Source: CAD feature listing. Evaluate the final solid. Frame: model axes, mm. A direction names the side the tool comes from. Round coordinates to 2 decimals unless told otherwise and drop trailing zeros. Order: outer loops, then holes, each group sorted by start corner. A loop starts at its lowest first (then second) coordinate and runs counter-clockwise, first axis right, second up. Notation, with made-up numbers: (-33.75, -22) -> (-5.75, -22) arc R17 cw to (-5.75, -6) -> close; hole circle Ø4 at (41, 44.5). An arc over 180 degrees is marked (long way). Use a Markdown table: item, result. Add a question column.
```python
from build123d import *

# Parameters (mm, degrees)
SKETCH_1_R               = 8
EXTRUDE_1_DEPTH          = 180
SKETCH_2_R               = 4
CUT_EXTRUDE_1_DEPTH      = 9
CUT_EXTRUDE_1_DEPTH_BACK = 9
SKETCH_3_OUTSIDE_W       = 54.284
SKETCH_3_OUTSIDE_H       = 54.284
SKETCH_3_OUTSIDE_W_2     = 8
SKETCH_3_OUTSIDE_H_2     = 20
CUT_EXTRUDE_2_DEPTH      = 20


with BuildPart() as part:
    # 草图1 → 凸台-拉伸1 (new body)
    with BuildSketch(Plane(origin=(0, 0, 0), x_dir=(0, 0, -1), z_dir=(1, 0, 0))):
        Circle(SKETCH_1_R)
    extrude(amount=EXTRUDE_1_DEPTH)

    # 草图2 → 切除-拉伸1 (cut, two sides)
    with BuildSketch(Plane.XY) as cut_extrude_1_sk:
        with Locations((10, 0)):
            Circle(SKETCH_2_R)
        with Locations((170, 0)):
            Circle(SKETCH_2_R)
    extrude(amount=CUT_EXTRUDE_1_DEPTH, mode=Mode.SUBTRACT)
    extrude(cut_extrude_1_sk.sketch, amount=-CUT_EXTRUDE_1_DEPTH_BACK, mode=Mode.SUBTRACT)

    # 草图3 outside → 切除-拉伸2 (cut)
    with BuildSketch(Plane.ZY):
        Rectangle(SKETCH_3_OUTSIDE_W, SKETCH_3_OUTSIDE_H)
        Rectangle(SKETCH_3_OUTSIDE_W_2, SKETCH_3_OUTSIDE_H_2, mode=Mode.SUBTRACT)
    extrude(amount=-CUT_EXTRUDE_2_DEPTH, mode=Mode.SUBTRACT)


solid = part.part
```
1) Line query: probe 1 along X at (y, z) = (0, 4.75); probe 2 along X at (y, z) = (3.5, 1.75); probe 3 along X at (y, z) = (-2, -2). Output: solid intervals per line, ascending. Write a range as from..to.
2) Section A-A on y = 0. Output: boundary loops of the cut face in (x, z), then the cut area to 3 significant figures.
3) Section B-B on x = 10. Output: boundary loops of the cut face in (y, z), then the cut area to 3 significant figures.
4) Reachability of faces 1 (the flat face through (20, 0, 6)), 2 (the flat face through (180, 0, 0)) from +Z, -Z, +X, -X, +Y, -Y: full face, straight path, thin tool, end or side. Return the list, or none.
5) Section D-D on x = 170. Output: boundary loops of the cut face in (y, z), then the cut area to 3 significant figures.
6) Section C-C on z = 0. Output: boundary loops of the cut face in (x, y), then the cut area to 3 significant figures.
7) First-contact query: pin 1 Ø5 at (x, y) = (10, 0) entering from +Z; pin 2 Ø3 at (x, y) = (52.5, -5.5) entering from -Z; pin 3 Ø6 at (x, y) = (142, -6) entering from -Z; pin 4 Ø4 at (x, y) = (7, 2.5) entering from -Z. Flat tips, straight axial feed; report the tip coordinate or a pass-through.
8) Draft query along X for faces 3 (the flat face through (5, 0, -4)), 4 (the flat face through (20, 0, -6)), 5 (the cylindrical face through (6, 0, 0)), 6 (the cylindrical face through (172.15, 3.373, 0.117)). Return one class per face: pulls with the +X half, pulls with the -X half, needs draft (parallel to the pull), parting line crosses it, or undercut.
Conclusion:
| question | item | result |
|---|---|---|
| 1 | probe 1 | x = 20..166, 174..180 |
| 1 | probe 2 | x = 0..8.06, 11.94..168.06, 171.94..180 |
| 1 | probe 3 | x = 0..6.54, 13.46..166.54, 173.46..180 |
| 2 | outline | (0, -4) -> (6, -4) -> (6, 4) -> (0, 4) -> close; (14, -4) -> (20, -4) -> (20, -8) -> (166, -8) -> (166, 8) -> (20, 8) -> (20, 4) -> (14, 4) -> close; (174, -8) -> (180, -8) -> (180, 8) -> (174, 8) -> close |
| 2 | area | 2,530 mm^2 |
| 3 | outline | (-6.93, -4) -> (-4, -4) -> (-4, 4) -> (-6.93, 4) arc R8 ccw to start; (4, -4) -> (6.93, -4) arc R8 ccw to (6.93, 4) -> (4, 4) -> close |
| 3 | area | 58.4 mm^2 |
| 4 | face 1 | +Z, -X, +Y, -Y |
| 4 | face 2 | +Z, -Z, +X, +Y, -Y |
| 5 | outline | (-4, -6.93) -> (-4, 6.93) arc R8 ccw to start; (4, -6.93) arc R8 ccw to (4, 6.93) -> close |
| 5 | area | 78.6 mm^2 |
| 6 | outline | (0, -8) -> (180, -8) -> (180, 8) -> (0, 8) -> close; hole circle Ø8 at (10, 0); hole circle Ø8 at (170, 0) |
| 6 | area | 2,780 mm^2 |
| 7 | pin 1 | passes through |
| 7 | pin 2 | stops at z = -6.93 |
| 7 | pin 3 | stops at z = -7.42 |
| 7 | pin 4 | stops at z = -4 |
| 8 | face 3 | needs draft |
| 8 | face 4 | pulls with the -X half |
| 8 | face 5 | undercut |
| 8 | face 6 | undercut |
